Verification items for the finished model (mm, model axes). A direction names the side the tool comes from. Round coordinates to 2 decimals unless told otherwise and drop trailing zeros. Write each loop counter-clockwise with the first axis right and the second up, starting at its lowest first coordinate (ties: lowest second). Pieces come first, ordered by that corner, then holes. Notation, with made-up numbers: M 32.25,68 L 84.25,68 A16 cw 84.25,79 Z; hole C 25.5,30 d9. An arc over 180 degrees is marked long. Answer in a Markdown table with one row per item. Add a question column.
1. Sectioned sample at A-A on y = 30. Record the cut outline in (x, z).
2. Draft check along Y on faces 1 (the flat face through (0, 82, 3)), 2 (the flat face through (124, 38.1, 3)), 3 (the flat face through (3, 12.7, 3)), 4 (the flat face through (111, 95.25, 3)). Enter one of: pulls with the +Y half, pulls with the -Y half, needs draft (parallel to the pull), parting line crosses it, or undercut.
3. Material ranges on probe 1 along Y at (x, z) = (63.5, 3); probe 2 along X at (y, z) = (88, 3.5); probe 3 along X at (y, z) = (79, 1.25), recorded low to high.
4. Set-up check for faces 5 (the flat face through (127, 32, 3)), 6 (the flat face through (25.4, 32, 3)), 7 (the flat face through (6.35, 19, 3)), 8 (the flat face through (124, 50.8, 3)), 9 (the flat face through (3, 88.9, 3)): record each of +Z, -Z, +X, -X, +Y, -Y from which the full face is reachable in a straight line by a thin tool's end or side.
5. Sectioned sample at C-C on z = 1.5. Count the separate pieces of the cut face and the enclosed holes in it, plus the area to 3 significant figures.
6. Sectioned sample at B-B on x = 63.5. Record the cut outline in (y, z), plus the area to 3 significant figures.
7. Sectioned sample at D-D on x = 80.5. Record the cut outline in (y, z).
8. Go/stop test with flat-tipped pins: pin 1 Ø3 at (y, z) = (20.5, 3) entering from -X; pin 2 Ø1.9 at (x, z) = (3, 2) entering from +Y. Record where each tip stops, or that it passes through.
```python
from build123d import *

# Parameters (mm, degrees)
SKETCH1_W           = 127
SKETCH1_H           = 95.25
BOSS_EXTRUDE1_DEPTH = 6.35
SKETCH2_R           = 3.96875
CUT_EXTRUDE1_DEPTH  = 7.35
SKETCH3_W           = 6.35
SKETCH3_H           = 12.7
CUT_EXTRUDE2_DEPTH  = 7.35
SKETCH4_W           = 6.35
SKETCH4_H           = 12.7
CUT_EXTRUDE3_DEPTH  = 7.35
LPATTERN1_COUNT     = 4
LPATTERN1_PITCH     = 25.4
CUT_EXTRUDE4_DEPTH  = 7.35


with BuildPart() as part:
    # Sketch1 → Boss-Extrude1 (new body)
    with BuildSketch(Plane.XY):
        with Locations((63.5, 47.625)):
            Rectangle(SKETCH1_W, SKETCH1_H)
    extrude(amount=BOSS_EXTRUDE1_DEPTH)

    # Sketch2 → Cut-Extrude1 (cut, through all)
    with BuildSketch(Plane.XY.offset(6.35)):
        with Locations((63.5, 38.1)):
            Circle(SKETCH2_R)
    extrude(amount=-CUT_EXTRUDE1_DEPTH, mode=Mode.SUBTRACT)

    # Sketch3 → Cut-Extrude2 (cut, through all)
    with BuildSketch(Plane.XY.offset(6.35)):
        with Locations((3.175, 19.05)):
            Rectangle(SKETCH3_W, SKETCH3_H)
    cut_extrude2 = extrude(amount=-CUT_EXTRUDE2_DEPTH, mode=Mode.SUBTRACT)

    # Sketch4 → Cut-Extrude3 (cut, through all)
    with BuildSketch(Plane.XY.offset(6.35)):
        with Locations((123.825, 19.05)):
            Rectangle(SKETCH4_W, SKETCH4_H)
    cut_extrude3 = extrude(amount=-CUT_EXTRUDE3_DEPTH, mode=Mode.SUBTRACT)

    # LPattern1: Cut-Extrude2, Cut-Extrude3 ×4
    with Locations(*[(0, i * LPATTERN1_PITCH, 0) for i in range(1, LPATTERN1_COUNT)]):
        add(cut_extrude2, mode=Mode.SUBTRACT)
        add(cut_extrude3, mode=Mode.SUBTRACT)

    # Sketch5 → Cut-Extrude4 (cut, through all)
    with BuildSketch(Plane.XY.offset(6.35)):
        Polygon((25.4, 95.25), (25.4, 82.094090512), (101.6, 38.1), (101.6, 95.25), align=None)
        Polygon((25.4, 38.1), (47.397045256, 25.4), (25.4, 25.4), align=None)
    extrude(amount=-CUT_EXTRUDE4_DEPTH, mode=Mode.SUBTRACT)


solid = part.part
```
Geometry check:
| question | item | result |
|---|---|---|
| 1 | outline | M 0,0 L 25.4,0 L 25.4,6.35 L 0,6.35 Z; M 39.43,0 L 127,0 L 127,6.35 L 39.43,6.35 Z |
| 2 | face 1 | needs draft |
| 2 | face 2 | undercut |
| 2 | face 3 | undercut |
| 2 | face 4 | pulls with the +Y half |
| 3 | probe 1 | y = 0 to 34.13, 42.07 to 60.1 |
| 3 | probe 2 | x = 0 to 25.4, 101.6 to 127 |
| 3 | probe 3 | x = 0 to 30.76, 101.6 to 127 |
| 4 | face 5 | +Z, -Z, +X, +Y, -Y |
| 4 | face 6 | +Z, -Z |
| 4 | face 7 | +Z, -Z, -X |
| 4 | face 8 | +Z, -Z, +X |
| 4 | face 9 | +Z, -Z, -X, +Y |
| 5 | separate pieces | 1 |
| 5 | enclosed holes | 2 |
| 5 | area | 8,660 mm2 |
| 6 | outline | M 0,0 L 34.13,0 L 34.13,6.35 L 0,6.35 Z; M 42.07,0 L 60.1,0 L 60.1,6.35 L 42.07,6.35 Z |
| 6 | area | 331 mm2 |
| 7 | outline | M 0,0 L 50.28,0 L 50.28,6.35 L 0,6.35 Z |
| 8 | pin 1 | stops at x = 6.35 |
| 8 | pin 2 | stops at y = 88.9 |
